Check sheet for the drawn part. Datum: minimum x, y, z corner. Units: mm. A direction names the side the tool comes from. Round coordinates to 2 decimals unless told otherwise and drop trailing zeros. Loops run counter-clockwise (first coordinate to the right, second up) from the corner with the lowest first, then second, coordinate; pieces in that order, holes last.
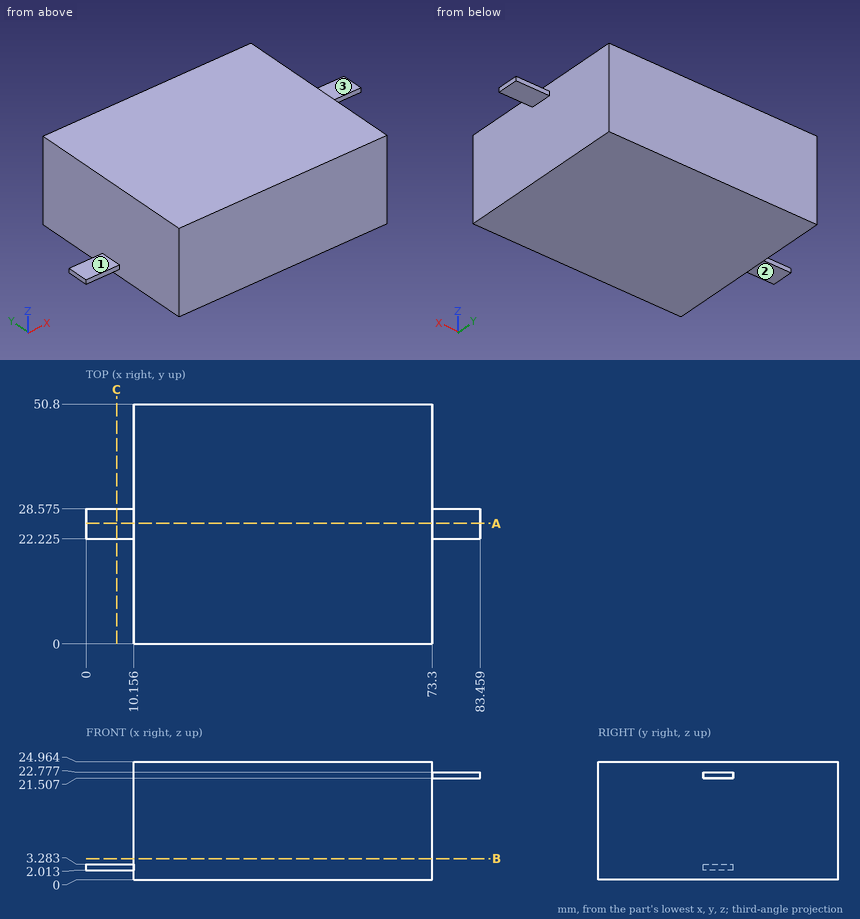
1) Gauge pin test, flat ends, axial feed: pin 1 (1.5 mm diameter, centred on x = 63, z = 6.5, fed in from -Y); pin 2 (5 mm diameter, centred on x = 78.5, y = 24, fed in from +Z); pin 3 (5 mm diameter, centred on x = 3.5, y = 26.5, fed in from -Z); pin 4 (1 mm diameter, centred on y = 11, z = 12.5, fed in from -X). Record the tip position at first contact, or that the pin passes through.
Report:
pin 1: stops at y = 0
pin 2: stops at z = 22.78
pin 3: stops at z = 2.01
pin 4: stops at x = 10.16
2) Access from +Z, -Z, +X, -X, +Y, -Y to the whole of each face (thin tool, end or side, straight path). Record for the marked faces 1, 2 and 3.
Report:
face 1: +Z, -X, +Y, -Y
face 2: -Z, -X, +Y, -Y
face 3: +Z, +X, +Y, -Y
3) Sectioned sample at A-A, the plane y = 25.5. Record the cut outline in (x, z) (1 decimal).
Report:
outline: (0, 2) - (10.2, 2) - (10.2, 0) - (73.3, 0) - (73.3, 21.5) - (83.5, 21.5) - (83.5, 22.8) - (73.3, 22.8) - (73.3, 25) - (10.2, 25) - (10.2, 3.3) - (0, 3.3) - close
4) Sectioned sample at C-C, the plane x = 6.5. Record the cut outline in (y, z) (1 decimal).
Report:
outline: (22.2, 2) - (28.6, 2) - (28.6, 3.3) - (22.2, 3.3) - close
5) Scan line: line 1 along X through (y, z) = (8, 14) (1 decimal). Record every from-to range of solid material in increasing order.
Report:
line 1: x = 10.2 to 73.3
6) Sectioned sample at B-B, the plane z = 4.5. Record the cut outline in (x, y) (1 decimal), then the cut area to 3 significant figures.
Report:
outline: (10.2, 0) - (73.3, 0) - (73.3, 50.8) - (10.2, 50.8) - close
area: 3,210 mm2
